The model under review builds one solid part; all positions refer to its coordinate system, in mm. Face numbers are marked on the shaded views. A direction names the side the tool comes from. Round coordinates to 2 decimals unless told otherwise and drop trailing zeros. Order: outer loops, then holes, each group sorted by start corner. A loop starts at its lowest first (then second) coordinate and runs counter-clockwise, first axis right, second up. Notation, with made-up numbers: (29.25, 59.25) - (36.25, 59.25) arc R15 ccw to (36.25, 65.25) - close; hole circle Ø9 at (71.25, -33.75). An arc over 180 degrees is marked (long way). One line per question, with ' | ' between items. Start each with the question number.
Item 1: Add section B-B on z = 5. State the section outline as (x, y) points (3 decimals), and give its area (3 significant figures).
Item 2: Tool access review of the marked faces 1, 2 and 3: name each direction out of +Z, -Z, +X, -X, +Y, -Y from which nothing blocks a thin tool from reaching the whole face with its end or side.
Item 3: For L1, parallel to Y at x = 3, z = 1.5; L2, parallel to X at y = 1.5, z = 2.5; L3, parallel to X at y = 8.5, z = 3, list the stretches that pass through material, from the lowest coordinate up. Write a range as [from, to].
Item 4: Insertion check: pin 1 Ø4.5 at (x, y) = (0, 21) entering from +Z; pin 2 Ø6.5 at (x, y) = (0, 0) entering from -Z; pin 3 Ø1.2 at (x, z) = (-0.5, 2.5) entering from +Y; pin 4 Ø4 at (y, z) = (1, 5.5) entering from -X. Each pin has a flat end and moves straight along its axis. Give the tip position at first contact, or say it passes through.
Item 5: Add section A-A on y = 0. State the section outline as (x, z) points (3 decimals), and give its area (3 significant figures).
Item 6: Add section C-C on x = -1. State how many separate pieces and enclosed holes the cut face has, and give its area (3 significant figures).
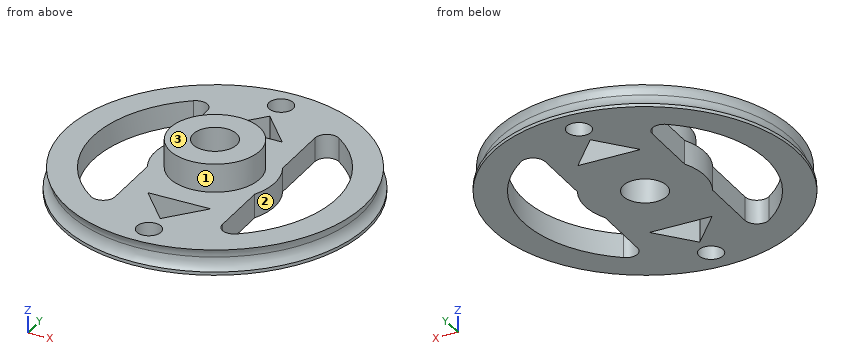
from build123d import *

# Parameters (mm, degrees)
F0_R     = 25.4
F0_R_2   = 3.625
F1_DEPTH = 4
F2_R     = 7.5
F2_R_2   = 3.625
F3_DEPTH = 4.75
F4_R     = 2.020962
F5_DEPTH = 4.001
F6_R     = 2.5


with BuildPart() as f1:
    # F0 (on Top) → F1 (new body)
    with BuildSketch(Plane.XY):
        Circle(F0_R)
        with BuildLine():
            Line((-8.950036, 14.687379), (-8.950036, 4.46059))
            ThreePointArc((-8.950036, 4.46059), (-10, 0), (-8.950036, -4.46059))
            Line((-8.950036, -4.46059), (-8.950036, -14.687379))
            ThreePointArc((-8.950036, -14.687379), (-10.053051, -16.474953), (-12.145455, -16.290805))
            ThreePointArc((-12.145455, -16.290805), (-20.32, 0), (-12.145455, 16.290805))
            ThreePointArc((-12.145455, 16.290805), (-10.053051, 16.474953), (-8.950036, 14.687379))
        make_face(mode=Mode.SUBTRACT)
        Circle(F0_R_2, mode=Mode.SUBTRACT)
        with BuildLine():
            Line((8.950036, 4.46059), (8.950036, 14.687379))
            ThreePointArc((8.950036, 14.687379), (10.053051, 16.474953), (12.145455, 16.290805))
            ThreePointArc((12.145455, 16.290805), (20.32, 0), (12.145455, -16.290805))
            ThreePointArc((12.145455, -16.290805), (10.053051, -16.474953), (8.950036, -14.687379))
            Line((8.950036, -14.687379), (8.950036, -4.46059))
            ThreePointArc((8.950036, -4.46059), (10, 0), (8.950036, 4.46059))
        make_face(mode=Mode.SUBTRACT)
    extrude(amount=F1_DEPTH)

    # F2 (on face) → F3 (join)
    with BuildSketch(Plane.XY.offset(4)):
        Circle(F2_R)
        Circle(F2_R_2, mode=Mode.SUBTRACT)
    extrude(amount=F3_DEPTH)

    # F4 (on face) → F5 (cut, through all)
    with BuildSketch(Plane.XY.offset(4)):
        Polygon((-5.234685, 11.362989), (0, 11.362989), (0, 17.41166), align=None)
        Polygon((0, 17.41166), (0, 11.362989), (5.234685, 11.362989), align=None)
        Polygon((0, -11.362989), (-5.234685, -11.362989), (0, -17.41166), (5.234685, -11.362989), align=None)
        with Locations((0, 20.997725)):
            Circle(F4_R)
        with Locations((0, -20.997725)):
            Circle(F4_R)
    extrude(amount=-F5_DEPTH, mode=Mode.SUBTRACT)

    # F6 (on Front) → F7 (revolve, cut)
    with BuildSketch(Plane.XZ):
        with Locations((-26.922889, 2.530067)):
            Circle(F6_R)
    revolve(axis=Axis((0, 0, 7.021954), (0, 0, -1)), mode=Mode.SUBTRACT)


solid = f1.part
Determined:
1) outline: circle Ø15 at (0, 0); hole circle Ø7.25 at (0, 0) | area: 135 mm2
2) face 1: +Z | face 2: +Z, -Z | face 3: +Z, +X, -X, +Y, -Y
3) L1: [-24.46, -13.95], [-11.36, -2.03], [2.03, 11.36], [13.95, 24.46] | L2: [-24.38, -20.26], [-9.89, -3.3], [3.3, 9.89], [20.26, 24.38] | L3: [-22.94, -18.46], [-8.95, 8.95], [18.46, 22.94]
4) pin 1: z = 4 | pin 2: through | pin 3: y = 24.5 | pin 4: x = -24.9
5) outline: (-25.4, 0) - (-20.32, 0) - (-20.32, 4) - (-24.901, 4) arc R2.5 cw to (-25.4, 0.547) - close; (-10, 0) - (-3.625, 0) - (-3.625, 8.75) - (-7.5, 8.75) - (-7.5, 4) - (-10, 4) - close; (3.625, 0) - (10, 0) - (10, 4) - (7.5, 4) - (7.5, 8.75) - (3.625, 8.75) - close; (20.32, 0) - (25.4, 0) - (25.4, 0.547) arc R2.5 cw to (24.901, 4) - (20.32, 4) - close | area: 123 mm2
6) separate pieces: 6 | enclosed holes: 0 | area: 140 mm2
